Drawing for the job (mm, zero at the part's lowest x, y, z). A direction names the side the tool comes from. Coordinates: 2 decimals unless noted, no trailing zeros. Loops run counter-clockwise (first coordinate to the right, second up) from the corner with the lowest first, then second, coordinate; pieces in that order, holes last. Notation, with made-up numbers: (48.5, 56) -> (52.5, 56) arc R15 cw to (52.5, 74) -> close; hole circle Ø4 at (-9.5, 62). An arc over 180 degrees is marked (long way). Write item = value, one per line. Start each with the question number.
(1) Tool access for the marked faces 1, 2, 3 and 4: list every direction of +Z, -Z, +X, -X, +Y, -Y with a clear straight run to the whole face (end or side of a thin tool).
(2) Band-saw the part on A-A (x = 8). Write the cut outline in (y, z).
(3) Flat gauge pins, fed straight in: P1, Ø1, axis at y = 10, z = 10, coming from the -X side; P2, Ø1.5, axis at x = 5.5, z = 30.5, coming from the +Y side; P3, Ø5, axis at x = 9, y = 4.5, coming from the -Z side; P4, Ø6, axis at x = 9.5, z = 6, coming from the -Y side. Where does each tip first touch, or does it go through?
(4) Band-saw the part on D-D (z = 19). Write the cut outline in (x, y).
(5) Band-saw the part on C-C (z = 10.5). Write the cut outline in (x, y).
(6) Drill centre lines: line 1 (Z direction, x = 4.75, y = 14.5); line 2 (Z direction, x = 6, y = 12.75); line 3 (Y direction, x = 6, z = 26) (1 decimal). Where is each one in solid material? Low to high. Write a range as from..to.
(7) Band-saw the part on B-B (y = 8). Write the cut outline in (x, z), and give its area (3 significant figures).
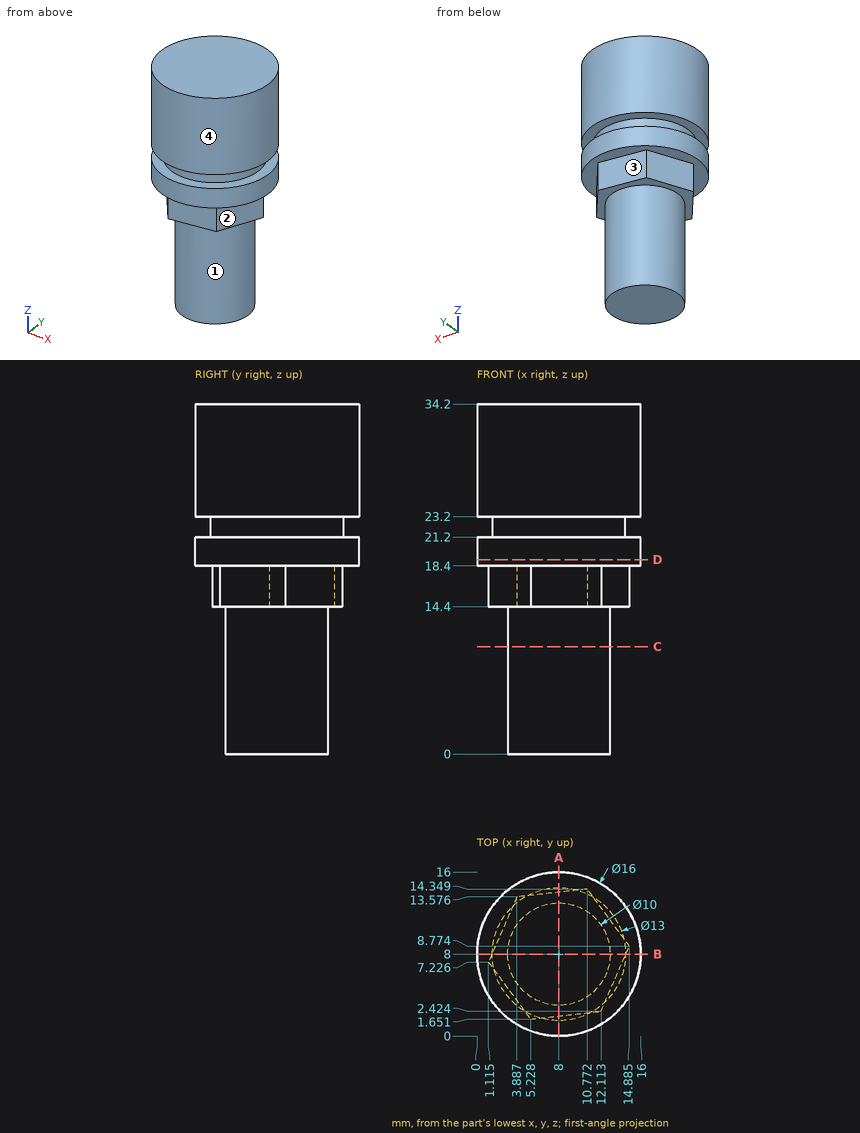
Findings below:
q1.face_1 = -Z
q1.face_2 = -Z, +X, -Y
q1.face_3 = -Z, -X, +Y
q1.face_4 = +Z, -Z
q2.outline = (0, 18.4) -> (1.96, 18.4) -> (1.96, 14.4) -> (3, 14.4) -> (3, 0) -> (13, 0) -> (13, 14.4) -> (14.04, 14.4) -> (14.04, 18.4) -> (16, 18.4) -> (16, 21.2) -> (14.5, 21.2) -> (14.5, 23.2) -> (16, 23.2) -> (16, 34.2) -> (0, 34.2) -> (0, 23.2) -> (1.5, 23.2) -> (1.5, 21.2) -> (0, 21.2) -> close
q3.P1 = 3.23
q3.P2 = 15.81
q3.P3 = 0
q3.P4 = 3
q4.outline = circle Ø16 at (8, 8)
q5.outline = circle Ø10 at (8, 8)
q6.line_1 = 18.4..21.2, 23.2..34.2
q6.line_2 = 14.4..34.2
q6.line_3 = 0.3..15.7
q7.outline = (0, 18.4) -> (1.45, 18.4) -> (1.45, 14.4) -> (3, 14.4) -> (3, 0) -> (13, 0) -> (13, 14.4) -> (14.55, 14.4) -> (14.55, 18.4) -> (16, 18.4) -> (16, 21.2) -> (14.5, 21.2) -> (14.5, 23.2) -> (16, 23.2) -> (16, 34.2) -> (0, 34.2) -> (0, 23.2) -> (1.5, 23.2) -> (1.5, 21.2) -> (0, 21.2) -> close
q7.area = 443 mm²
